Part model, mm, in its own coordinate system. Coordinates: 2 decimals unless noted, no trailing zeros. Loops run counter-clockwise (first coordinate to the right, second up) from the corner with the lowest first, then second, coordinate; pieces in that order, holes last. Notation, with made-up numbers: (57, 31.5) -> (116, 31.5) arc R14 ccw to (116, 36.5) -> close; hole circle Ø3 at (31.5, 33). An arc over 180 degrees is marked (long way). One line per question, with ' | ' between items. Start each with the question number.
1) Cut at B-B (z = 18). List the corners of the cut face in (x, y), plus the area to 3 significant figures.
2) Cut at A-A (y = -2.25). List the corners of the cut face in (x, z) (1 decimal), plus the area to 3 significant figures.
3) Two-plate mould, pull along Z, no slides. Class faces 1 (the face through (40.56, -2.58, 8.2)), 2 (the face through (-214.24, -2.58, -48.29)), 3 (the face through (-214.24, -2.58, 63.43)): released by +Z, released by -Z, zero draft, split by the parting line, or undercut.
4) Probe L1, parallel to X at y = -2.1, z = 19; L2, parallel to Z at x = 68, y = -4.6; L3, parallel to Z at x = -170, y = -1. List the from-to ranges inside material, lowest first. Write a range as from..to.
from build123d import *

# Parameters (mm, degrees)
F0_W     = 322.58
F0_H     = 127
F1_DEPTH = 5.08
F2_R     = 25.4
F3_R     = 14.2875
F4_DEPTH = 25.4


with BuildPart() as f1:
    # F0 (on Front) → F1 (new body)
    with BuildSketch(Plane.XZ):
        with Locations((-60.191011, 7.567608)):
            Rectangle(F0_W, F0_H)
    extrude(amount=F1_DEPTH)

    # F2
    f2_edges = [f1.edges().sort_by_distance(p)[0] for p in [
        (101.098989, -2.54, 71.067608),
        (101.098989, -2.54, -55.932392),
        (-221.481011, -2.54, 71.067608),
        (-221.481011, -2.54, -55.932392),
    ]]
    fillet(f2_edges, radius=F2_R)

    # F3 (on face) → F4 (cut)
    with BuildSketch(Plane.XZ.offset(5.08)):
        with Locations((-60.191011, 7.567608)):
            Circle(F3_R)
        with Locations((54.832889, 7.567608)):
            Circle(F3_R)
        with Locations((-175.214911, 7.567608)):
            Circle(F3_R)
    extrude(amount=-F4_DEPTH, mode=Mode.SUBTRACT)


solid = f1.part
Reported:
1) outline: (-221.48, -5.08) -> (-184.98, -5.08) -> (-184.98, 0) -> (-221.48, 0) -> close; (-165.45, -5.08) -> (-69.95, -5.08) -> (-69.95, 0) -> (-165.45, 0) -> close; (-50.43, -5.08) -> (45.07, -5.08) -> (45.07, 0) -> (-50.43, 0) -> close; (64.59, -5.08) -> (101.1, -5.08) -> (101.1, 0) -> (64.59, 0) -> close | area: 1,340 mm²
2) outline: (-221.5, -30.5) arc R25.4 ccw to (-196.1, -55.9) -> (75.7, -55.9) arc R25.4 ccw to (101.1, -30.5) -> (101.1, 45.7) arc R25.4 ccw to (75.7, 71.1) -> (-196.1, 71.1) arc R25.4 ccw to (-221.5, 45.7) -> close; hole circle Ø28.6 at (-175.2, 7.6); hole circle Ø28.6 at (-60.2, 7.6); hole circle Ø28.6 at (54.8, 7.6) | area: 38,500 mm²
3) face 1: undercut | face 2: released by -Z | face 3: released by +Z
4) L1: x = -221.48..-183.78, -166.65..-68.76, -51.62..46.26, 63.4..101.1 | L2: z = -55.93..2.02, 13.11..71.07 | L3: z = -55.93..-5.73, 20.87..71.07
